```python
from build123d import *

# Parameters (mm, degrees)
SKETCH1_W           = 47
SKETCH1_H           = 69
BOSS_EXTRUDE1_DEPTH = 2
FILLET1_R           = 7
SKETCH2_W           = 20
SKETCH2_H           = 14
SKETCH2_H_2         = 21.8
CUT_EXTRUDE1_DEPTH  = 2
SKETCH3_W           = 3.5
SKETCH3_H           = 19.5
BOSS_EXTRUDE2_DEPTH = 6
FILLET2_R           = 4
FILLET3_R           = 2.5
SKETCH4_R           = 1
CUT_EXTRUDE2_DEPTH  = 444.714975323


with BuildPart() as part:
    # Sketch1 → Boss-Extrude1 (new body)
    with BuildSketch(Plane.XY.offset(10)):
        with Locations((-239.856711142, 406.898341584)):
            Rectangle(SKETCH1_W, SKETCH1_H)
    extrude(amount=BOSS_EXTRUDE1_DEPTH)

    # Fillet1
    fillet1_edges = [part.edges().sort_by_distance(p)[0] for p in [
        (-263.356711142, 441.398341584, 11),
        (-216.356711142, 441.398341584, 11),
        (-216.356711142, 372.398341584, 11),
        (-263.356711142, 372.398341584, 11),
    ]]
    fillet(fillet1_edges, radius=FILLET1_R)

    # Sketch2 → Cut-Extrude1 (cut)
    with BuildSketch(Plane.XY.offset(12)):
        with Locations((-237.923586614, 425.007047567)):
            Rectangle(SKETCH2_W, SKETCH2_H)
        with Locations((-237.923586614, 394.052620238)):
            Rectangle(SKETCH2_W, SKETCH2_H_2)
    extrude(amount=-CUT_EXTRUDE1_DEPTH, mode=Mode.SUBTRACT)

    # Sketch3 → Boss-Extrude2 (add)
    with BuildSketch(Plane.XY.offset(12)):
        with Locations((-220.053070068, 411.047943115)):
            Rectangle(SKETCH3_W, SKETCH3_H)
        with Locations((-256.157684326, 411.411865234)):
            Rectangle(SKETCH3_W, SKETCH3_H)
    extrude(amount=BOSS_EXTRUDE2_DEPTH)

    # Fillet2
    fillet2_edges = [part.edges().sort_by_distance(p)[0] for p in [
        (-247.923586614, 418.007047567, 11),
        (-247.923586614, 432.007047567, 11),
        (-227.923586614, 432.007047567, 11),
        (-227.923586614, 418.007047567, 11),
        (-247.923586614, 383.152620238, 11),
        (-247.923586614, 404.952620238, 11),
        (-227.923586614, 404.952620238, 11),
        (-227.923586614, 383.152620238, 11),
    ]]
    fillet(fillet2_edges, radius=FILLET2_R)

    # Fillet3
    fillet3_edges = [part.edges().sort_by_distance(p)[0] for p in [
        (-256.157684326, 421.161865234, 12),
        (-256.157684326, 401.661865234, 12),
        (-256.157684326, 421.161865234, 18),
        (-256.157684326, 401.661865234, 18),
        (-220.053070068, 401.297943115, 12),
        (-220.053070068, 420.797943115, 12),
        (-220.053070068, 401.297943115, 18),
        (-220.053070068, 420.797943115, 18),
    ]]
    fillet(fillet3_edges, radius=FILLET3_R)

    # Sketch4 → Cut-Extrude2 (cut, through all)
    with BuildSketch(Plane.ZY.offset(257.907684326)):
        with Locations((14.979375571, 415.479440957)):
            Circle(SKETCH4_R)
        with Locations((14.978983816, 407.479440966)):
            Circle(SKETCH4_R)
    extrude(amount=-CUT_EXTRUDE2_DEPTH, mode=Mode.SUBTRACT)


solid = part.part
```
Input: part model. Units: mm. Frame: model coordinates. A direction names the side the tool comes from. Coordinates: 2 decimals unless noted, no trailing zeros. Order: outer loops, then holes, each group sorted by start corner. A loop starts at its lowest first (then second) coordinate and runs counter-clockwise, first axis right, second up. Notation, with made-up numbers: (35, 72) - (75, 72) arc R30 ccw to (75, 100) - close; hole circle Ø1 at (65.5, -34.75). An arc over 180 degrees is marked (long way). Put each result on its own line as item: value.
1. Cut plane D-D on y = 410.5. Return the cut outline in (x, z), then the cut area to 3 significant figures.
Report:
outline: (-263.36, 10) - (-216.36, 10) - (-216.36, 12) - (-218.3, 12) - (-218.3, 18) - (-221.8, 18) - (-221.8, 12) - (-254.41, 12) - (-254.41, 18) - (-257.91, 18) - (-257.91, 12) - (-263.36, 12) - close
area: 136 mm2
2. Contact query for flat-ended pins moving along their axis: pin 1 Ø10 at (x, y) = (-247, 401) entering from +Z; pin 2 Ø1.1 at (x, z) = (-219.5, 15) entering from +Y; pin 3 Ø3 at (y, z) = (415.48, 14.98) entering from +X. Output: stop coordinate, or through.
Report:
pin 1: stops at z = 12
pin 2: stops at y = 420.8
pin 3: stops at x = -218.3
3. Reachability of faces 4 (the face through (-256.133, 400.91, 12.713)), 5 (the face through (-257.908, 411, 15)), 6 (the face through (-220.03, 421.55, 12.71)), 7 (the face through (-218.303, 411, 15)), 8 (the face through (-246.72, 403.81, 10.99)) from +Z, -Z, +X, -X, +Y, -Y: full face, straight path, thin tool, end or side. Return the list, or none.
Report:
face 4: +Z, -X, -Y
face 5: +Z, -X, +Y, -Y
face 6: +Z, +X, +Y
face 7: +Z, +X, +Y, -Y
face 8: +Z, -Z
4. Draft query along Y for faces 1 (the face through (-220.08, 408.47, 14.85)), 2 (the face through (-263.357, 407, 11)), 3 (the face through (-220.03, 402.01, 17.25)). Return one class per face: pulls with the +Y half, pulls with the -Y half, needs draft (parallel to the pull), parting line crosses it, or undercut.
Report:
face 1: undercut
face 2: needs draft
face 3: pulls with the -Y half
5. Cut plane B-B on y = 389. Return the cut outline in (x, z), then the cut area to 3 significant figures.
Report:
outline: (-263.36, 10) - (-247.92, 10) - (-247.92, 12) - (-263.36, 12) - close; (-227.92, 10) - (-216.36, 10) - (-216.36, 12) - (-227.92, 12) - close
area: 54.0 mm2
6. Line query: line 1 along Y through (x, z) = (-243.5, 10.75); line 2 along X through (y, z) = (420, 12.5); line 3 along Y through (x, z) = (-231, 11.5). Output: solid intervals per line, ascending.
Report:
line 1: y = 372.4 to 383.15, 404.95 to 418.01, 432.01 to 441.4
line 2: x = -257.91 to -254.41, -221.8 to -218.3
line 3: y = 372.4 to 383.26, 404.84 to 418.12, 431.9 to 441.4
7. Cut plane C-C on x = -238.5. Return the cut outline in (y, z), then the cut area to 3 significant figures.
Report:
outline: (372.4, 10) - (383.15, 10) - (383.15, 12) - (372.4, 12) - close; (404.95, 10) - (418.01, 10) - (418.01, 12) - (404.95, 12) - close; (432.01, 10) - (441.4, 10) - (441.4, 12) - (432.01, 12) - close
area: 66.4 mm2
8. Cut plane A-A on z = 11.25. Return the cut outline in (x, y).
Report:
outline: (-263.36, 379.4) arc R7 ccw to (-256.36, 372.4) - (-223.36, 372.4) arc R7 ccw to (-216.36, 379.4) - (-216.36, 434.4) arc R7 ccw to (-223.36, 441.4) - (-256.36, 441.4) arc R7 ccw to (-263.36, 434.4) - close; hole (-247.92, 387.15) arc R4 ccw to (-243.92, 383.15) - (-231.92, 383.15) arc R4 ccw to (-227.92, 387.15) - (-227.92, 400.95) arc R4 ccw to (-231.92, 404.95) - (-243.92, 404.95) arc R4 ccw to (-247.92, 400.95) - close; hole (-247.92, 422.01) arc R4 ccw to (-243.92, 418.01) - (-231.92, 418.01) arc R4 ccw to (-227.92, 422.01) - (-227.92, 428.01) arc R4 ccw to (-231.92, 432.01) - (-243.92, 432.01) arc R4 ccw to (-247.92, 428.01) - close
